Could you check a few things on this model? Use its own coordinates, in mm. A direction names the side the tool comes from. Round coordinates to 2 decimals unless told otherwise and drop trailing zeros. Order: outer loops, then holes, each group sorted by start corner. A loop starts at its lowest first (then second) coordinate and runs counter-clockwise, first axis right, second up. Notation, with made-up numbers: (-17.75, 40.25) - (25.25, 40.25) arc R11 ccw to (25.25, 61.25) - close; hole circle Ø9 at (70.25, 51). An arc over 180 degrees is marked (long way). Return JSON: item names as keys, results as strings. Group by question number.
from build123d import *

# Parameters (mm, degrees)
BOSS_EXTRUDE1_DEPTH  = 3
M3_CLEARANCE_HOLE1_D = 3.4
SKETCH2_OUTSIDE_W    = 168.672
SKETCH2_OUTSIDE_H    = 102.608
CUT_EXTRUDE1_DEPTH   = 10


with BuildPart() as part:
    # Sketch1 → Boss-Extrude1 (new body)
    with BuildSketch(Plane.XY):
        with BuildLine():
            Line((-93.536600288, 73.798841742), (22.52665856, 73.798841742))
            ThreePointArc((22.52665856, 73.798841742), (29.597726372, 76.72777393), (32.52665856, 83.798841742))
            Line((32.52665856, 83.798841742), (32.52665856, 133.798841742))
            ThreePointArc((32.52665856, 133.798841742), (29.597726372, 140.869909554), (22.52665856, 143.798841742))
            Line((22.52665856, 143.798841742), (-93.536600288, 143.798841742))
            ThreePointArc((-93.536600288, 143.798841742), (-100.6076681, 140.869909554), (-103.536600288, 133.798841742))
            Line((-103.536600288, 133.798841742), (-103.536600288, 83.798841742))
            ThreePointArc((-103.536600288, 83.798841742), (-100.6076681, 76.72777393), (-93.536600288, 73.798841742))
        make_face()
        Polygon((7.241251279, 79.113754803), (7.241251279, 115.298841742), (25.200464445, 115.298841742), (25.200464445, 141.298841742), (-63.686125174, 141.298841742), (-63.686125174, 139.298841742), (-98, 139.298841742), (-98, 79.113754803), align=None, mode=Mode.SUBTRACT)
    extrude(amount=BOSS_EXTRUDE1_DEPTH)

    # M3 Clearance Hole1 (through all)
    with Locations(Plane(origin=(0, 0, 0), x_dir=(-1, 0, 0), z_dir=(0, 0, -1))):
        with Locations((-28.497536526, 136.798841742), (-28.497536526, 81.798841742)):
            Hole(M3_CLEARANCE_HOLE1_D / 2)

    # Sketch2 outside → Cut-Extrude1 (cut)
    with BuildSketch(Plane.XY.offset(3)):
        with Locations((-35.505, 108.799)):
            Rectangle(SKETCH2_OUTSIDE_W, SKETCH2_OUTSIDE_H)
        with BuildLine():
            Line((-98, 111.232980273), (-100.276015927, 111.232980273))
            Line((-100.276015927, 111.232980273), (-100.276015927, 110.181279495))
            ThreePointArc((-100.276015927, 110.181279495), (-100.885260547, 108.11074669), (-101.110575194, 110.257259772))
            Line((-101.110575194, 110.257259772), (-101.110575194, 111.232980273))
            Line((-101.110575194, 111.232980273), (-103.536600288, 111.232980273))
            Line((-103.536600288, 111.232980273), (-103.536600288, 155.169137996))
            Line((-103.536600288, 155.169137996), (37.520914888, 146.495442913))
            Line((37.520914888, 146.495442913), (36.419995989, 128.591552724))
            Line((36.419995989, 128.591552724), (32.52665856, 128.591552724))
            Line((32.52665856, 128.591552724), (29.357018022, 128.591552724))
            Line((29.357018022, 128.591552724), (29.357018022, 126.79555932))
            ThreePointArc((29.357018022, 126.79555932), (28.609769319, 124.402587901), (28.09640217, 126.856390462))
            Line((28.09640217, 126.856390462), (28.09640217, 128.591552724))
            Line((28.09640217, 128.591552724), (25.200464445, 128.591552724))
            Line((25.200464445, 128.591552724), (-98, 111.232980273))
        make_face(mode=Mode.SUBTRACT)
    extrude(amount=-CUT_EXTRUDE1_DEPTH, mode=Mode.SUBTRACT)


solid = part.part
1) I want a section at B-B, the plane z = 1. List the corners of the cut face in (x, y) for me, plus the area to 3 significant figures.
2) We'd pull the mould along Y, two halves only. Please class faces 1 (the flat face through (-19, 141.299, 1)), 2 (the flat face through (-98, 125, 1)), 3 (the cylindrical face through (29.411, 138.232, 1.521)): +Y half, -Y half, draft (parallel to the pull), parting line (faces both ways), or undercut.
3) I want a section at D-D, the plane y = 123. List the corners of the cut face in (x, z) for me.
4) If I drill on line 1 along X through (y, z) = (135.5, 2); line 2 along X through (y, z) = (130, 0.95); line 3 along X through (y, z) = (137, 0.7), over which ranges is the centre line in solid material (lowest first)? Write a range as from..to.
5) Will these pins go through, and if not, where does the flat tip stop? pin 1 (1.5 mm diameter, centred on x = -3, z = 1, fed in from -Y); pin 2 (0.9 mm diameter, centred on x = 26, z = 2, fed in from -Y); pin 3 (0.8 mm diameter, centred on y = 110.5, z = 1, fed in from -X).
6) I want a section at A-A, the plane y = 132. List the corners of the cut face in (x, z) for me, plus the area to 3 significant figures.
7) I want a section at C-C, the plane x = -16. List the corners of the cut face in (y, z) for me, plus the area to 3 significant figures.
8) For faces 4 (the flat face through (25.2, 135, 1)), 5 (the flat face through (-102, 111.233, 2)), 6 (the flat face through (-99, 111.233, 2)), which set-ups out of +Z, -Z, +X, -X, +Y, -Y let a thin tool reach every point of the face, with its end or its side?
Outcome:
{
 "1": {"outline": "(-103.54, 111.23) - (-101.11, 111.23) - (-101.11, 110.26) arc R1.1 ccw (long way) to (-100.28, 110.18) - (-100.28, 111.23) - (-98, 111.23) - (-98, 139.3) - (-63.69, 139.3) - (-63.69, 141.3) - (25.2, 141.3) - (25.2, 128.59) - (28.1, 128.59) - (28.1, 126.86) arc R1.3 ccw (long way) to (29.36, 126.8) - (29.36, 128.59) - (32.53, 128.59) - (32.53, 133.8) arc R10 ccw to (22.53, 143.8) - (-93.54, 143.8) arc R10 ccw to (-103.54, 133.8) - close; hole circle Ø3.4 at (28.5, 136.8)", "area": "628 mm^2"},
 "2": {"face 1": "-Y half", "face 2": "draft", "face 3": "undercut"},
 "3": {"outline": "(-103.54, 0) - (-98, 0) - (-98, 3) - (-103.54, 3) - close"},
 "4": {"line 1": "-103.39..-98, 25.2..27.4, 29.59..32.38", "line 2": "-103.54..-98, 25.2..32.53", "line 3": "-103.01..-98, 25.2..26.81, 30.19..32"},
 "5": {"pin 1": "y = 141.3", "pin 2": "y = 128.59", "pin 3": "x = -101.43"},
 "6": {"outline": "(-103.54, 0) - (-98, 0) - (-98, 3) - (-103.54, 3) - close; (25.2, 0) - (32.53, 0) - (32.53, 3) - (25.2, 3) - close", "area": "38.6 mm^2"},
 "7": {"outline": "(141.3, 0) - (143.8, 0) - (143.8, 3) - (141.3, 3) - close", "area": "7.50 mm^2"},
 "8": {"face 4": "+Z, -Z, -Y", "face 5": "+Z, -Z, -X", "face 6": "+Z, -Z, +X"}
}
